Geometry: see drawing. Coordinates: mm, zero at the bounding-box minimum. A direction names the side the tool comes from. Round coordinates to 2 decimals unless told otherwise and drop trailing zeros. Loops run counter-clockwise (first coordinate to the right, second up) from the corner with the lowest first, then second, coordinate; pieces in that order, holes last. Notation, with made-up numbers: (3, -1.5) - (7, -1.5) arc R22 cw to (7, 8.5) - close; hole circle Ø11 at (71, 29.25). An arc over 180 degrees is marked (long way). Write item = value, one per line. Start each with the question number.
Item 1: Line query: line 1 (Z direction, x = 58, y = 3); line 2 (X direction, y = 25.5, z = 8); line 3 (X direction, y = 5, z = 54.5). Output: solid intervals per line, ascending. Write a range as from..to.
Item 2: Section B-B (y = 2). Return loops of the section in (x, z), plus the area to 3 significant figures.
Item 3: Section D-D (y = 17.5). Return loops of the section in (x, z).
Item 4: Section A-A (x = 31.5). Return loops of the section in (y, z), plus the area to 3 significant figures.
Item 5: Access query for the marked faces 1, 2, 3 and 4. Directions: +Z, -Z, +X, -X, +Y, -Y. A direction counts if a zero-diameter tool reaches every point of the face in a straight line with its end or side. Return the directions, or none.
Item 6: First-contact query: pin 1 (3 mm diameter, centred on x = 22.5, z = 10, fed in from -Y); pin 2 (1.5 mm diameter, centred on y = 14.5, z = 34, fed in from +X); pin 3 (3 mm diameter, centred on x = 54, z = 45.5, fed in from +Y). Flat tips, straight axial feed; report the tip coordinate or a pass-through.
Item 7: Section C-C (z = 15). Return loops of the section in (x, y).
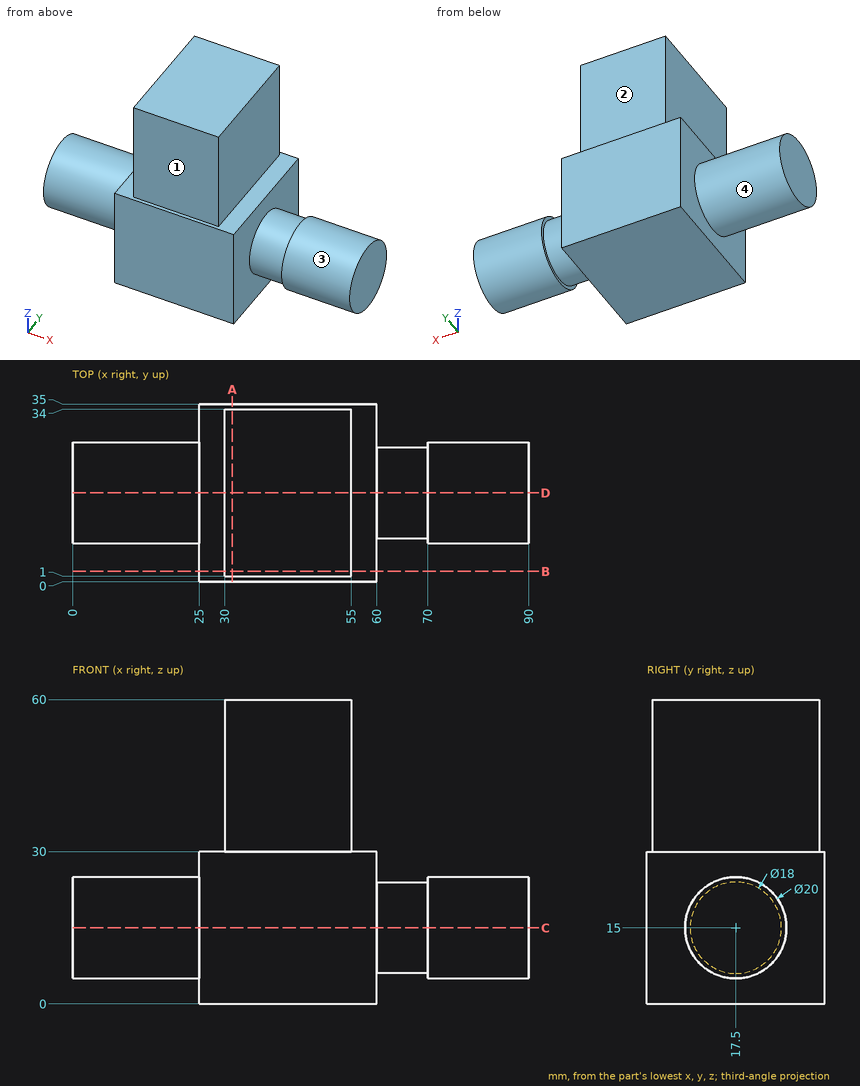
Taken from the geometry:
q1.line_1 = 0..30
q1.line_2 = 25..60
q1.line_3 = 30..55
q2.outline = (25, 0) - (60, 0) - (60, 30) - (55, 30) - (55, 60) - (30, 60) - (30, 30) - (25, 30) - close
q2.area = 1,800 mm^2
q3.outline = (0, 5) - (25, 5) - (25, 0) - (60, 0) - (60, 6) - (70, 6) - (70, 5) - (90, 5) - (90, 25) - (70, 25) - (70, 24) - (60, 24) - (60, 30) - (55, 30) - (55, 60) - (30, 60) - (30, 30) - (25, 30) - (25, 25) - (0, 25) - close
q4.outline = (0, 0) - (35, 0) - (35, 30) - (34, 30) - (34, 60) - (1, 60) - (1, 30) - (0, 30) - close
q4.area = 2,040 mm^2
q5.face_1 = +Z, +X, -X, -Y
q5.face_2 = +Z, +X, -X, +Y
q5.face_3 = +X
q5.face_4 = -X
q6.pin_1 = 8.13
q6.pin_2 = 55
q6.pin_3 = 34
q7.outline = (0, 7.5) - (25, 7.5) - (25, 0) - (60, 0) - (60, 8.5) - (70, 8.5) - (70, 7.5) - (90, 7.5) - (90, 27.5) - (70, 27.5) - (70, 26.5) - (60, 26.5) - (60, 35) - (25, 35) - (25, 27.5) - (0, 27.5) - close
